Input: part model. Units: mm. Frame: model coordinates. A direction names the side the tool comes from. Coordinates: 2 decimals unless noted, no trailing zeros. Write each loop counter-clockwise with the first axis right and the second up, starting at its lowest first coordinate (ties: lowest second). Pieces come first, ordered by that corner, then holes. Notation, with made-up numbers: (78, 60) - (102, 60) arc R18 ccw to (102, 77) - close; hole circle Ø5 at (-38, 89). An arc over 180 degrees is marked (long way). Put each result on its own line as item: value. Start each with the question number.
1. Access query for faces 1 (the cylindrical face through (5.44, -2.44, 0.54)), 2 (the flat face through (11.5, -0.5, 0.1)), 3 (the flat face through (12, 2, 0)). Directions: +Z, -Z, +X, -X, +Y, -Y. A direction counts if a zero-diameter tool reaches every point of the face in a straight line with its end or side. Return the directions, or none.
2. Line query: line 1 (Z direction, x = 1.25, y = 2); line 2 (Y direction, x = 11.25, z = 0); line 3 (X direction, y = -0.75, z = 1.75). Output: solid intervals per line, ascending.
3. Cut plane B-B, the plane y = 0. Return loops of the section in (x, z).
4. Cut plane A-A, the plane z = 0. Return loops of the section in (x, y).
5. Cut plane D-D, the plane x = 4.25. Return loops of the section in (y, z).
6. Pull-direction query (Y, two-part tool) for faces 4 (the conical face through (10.319, -1.08, -2.604)), 5 (the flat face through (11, 0, 0)), 6 (the flat face through (11.5, 0.5, 0.1)), 7 (the flat face through (12, -2, 0)); classes: released by +Y, released by -Y, zero draft, split by the parting line, or undercut.
7. Pin query (flat end, axial travel): pin 1 (3 mm diameter, centred on x = 3, z = 0, fed in from -Y); pin 2 (4 mm diameter, centred on x = 7, z = 2.5, fed in from +Y); pin 3 (1.5 mm diameter, centred on x = 2, y = -2, fed in from +Z). Return the tip coordinate at first contact, or that it passes through.
8. Cut plane C-C, the plane x = 10.25. Return loops of the section in (y, z).
from build123d import *

# Parameters (mm, degrees)
CHAMFER_1_SIZE      = 1
SKETCH_2_W          = 9.657524734
SKETCH_2_H          = 1
CUT_EXTRUDE_1_DEPTH = 1


with BuildPart() as part:
    # Эскиз1 → Повернуть1 (revolve)
    with BuildSketch(Plane(origin=(0, 0, 0), x_dir=(1, 0, 0), z_dir=(0, 1, 0))):
        Polygon((0, 0), (12, 0), (12, 4.5), (10, 2.5), (0, 2.5), align=None)
    revolve(axis=Axis((0, 0, 0), (1, 0, 0)))

    # Фаска1
    chamfer_1_edges = [part.edges().sort_by_distance(p)[0] for p in [
        (0, 0, 2.5),
    ]]
    chamfer(chamfer_1_edges, length=CHAMFER_1_SIZE)

    # Эскиз2 → Вырез-Вытянуть1 (cut)
    with BuildSketch(Plane(origin=(12, 0, 0), x_dir=(0, 0, -1), z_dir=(1, 0, 0))):
        Rectangle(SKETCH_2_W, SKETCH_2_H)
    extrude(amount=-CUT_EXTRUDE_1_DEPTH, mode=Mode.SUBTRACT)


solid = part.part
Report:
1. face 1: -X
1. face 2: +Z, -Z, +X
1. face 3: +Z, -Z, +X, +Y, -Y
2. line 1: z = -1.5 to 1.5
2. line 2: y = -3.75 to -0.5, 0.5 to 3.75
2. line 3: x = 0.4 to 12
3. outline: (0, -1.5) - (1, -2.5) - (10, -2.5) - (11, -3.5) - (11, 3.5) - (10, 2.5) - (1, 2.5) - (0, 1.5) - close
4. outline: (0, -1.5) - (1, -2.5) - (10, -2.5) - (12, -4.5) - (12, -0.5) - (11, -0.5) - (11, 0.5) - (12, 0.5) - (12, 4.5) - (10, 2.5) - (1, 2.5) - (0, 1.5) - close
5. outline: circle Ø5 at (0, 0)
6. face 4: split by the parting line
6. face 5: undercut
6. face 6: undercut
6. face 7: zero draft
7. pin 1: stops at y = -2.5
7. pin 2: stops at y = 2.45
7. pin 3: stops at z = 2.17
8. outline: circle Ø5.5 at (0, 0)
